from build123d import *

# Parameters (mm, degrees)
SKETCH1_W           = 40
SKETCH1_H           = 80
BOSS_EXTRUDE1_DEPTH = 100
CUT_EXTRUDE1_REACH  = 119.319
SKETCH3_W           = 40
SKETCH3_H           = 80
CUT_EXTRUDE2_REACH  = 119.319
SKETCH5_W           = 20
SKETCH5_H           = 40
CUT_EXTRUDE3_REACH  = 114.34
SKETCH6_R           = 12.5
CUT_EXTRUDE5_REACH  = 114.34


with BuildPart() as part:
    # Sketch1 → Boss-Extrude1 (new body)
    with BuildSketch(Plane(origin=(0, 0, 0), x_dir=(1, 0, 0), z_dir=(0, 1, 0))):
        with Locations((-1.364903769, -6.515993016)):
            Rectangle(SKETCH1_W, SKETCH1_H)
    extrude(amount=BOSS_EXTRUDE1_DEPTH)

    # Sketch3 → Cut-Extrude1 (cut, up to next)
    with BuildSketch(Plane(origin=(18.635096231, 0, 0), x_dir=(0, 0, -1), z_dir=(1, 0, 0)), mode=Mode.PRIVATE) as cut_extrude1_sk1:
        with Locations((-6.515993016, 60)):
            Rectangle(SKETCH3_W, SKETCH3_H)
    cut_extrude1_tool1 = extrude(cut_extrude1_sk1.sketch, amount=-CUT_EXTRUDE1_REACH, mode=Mode.PRIVATE) & part.part
    add(cut_extrude1_tool1.solids().sort_by_distance((18.635096, 60, 6.515993))[0], mode=Mode.SUBTRACT)

    # Sketch5 → Cut-Extrude2 (cut, up to next)
    with BuildSketch(Plane(origin=(18.635096231, 0, 0), x_dir=(0, 0, -1), z_dir=(1, 0, 0)), mode=Mode.PRIVATE) as cut_extrude2_sk1:
        with Locations((-36.515993016, 80)):
            Rectangle(SKETCH5_W, SKETCH5_H)
    cut_extrude2_tool1 = extrude(cut_extrude2_sk1.sketch, amount=-CUT_EXTRUDE2_REACH, mode=Mode.PRIVATE) & part.part
    add(cut_extrude2_tool1.solids().sort_by_distance((18.635096, 80, 36.515993))[0], mode=Mode.SUBTRACT)

    # Sketch6 → Cut-Extrude3 (cut, up to next)
    with BuildSketch(Plane.XZ, mode=Mode.PRIVATE) as cut_extrude3_sk1:
        with Locations((-1.364903769, 46.515993016)):
            Circle(SKETCH6_R)
    cut_extrude3_tool1 = extrude(cut_extrude3_sk1.sketch, amount=-CUT_EXTRUDE3_REACH, mode=Mode.PRIVATE) & part.part
    add(cut_extrude3_tool1.solids().sort_by_distance((-1.364904, 0, 46.515993))[0], mode=Mode.SUBTRACT)

    # Sketch10 → Cut-Extrude5 (cut, up to next)
    with BuildSketch(Plane.XZ, mode=Mode.PRIVATE) as cut_extrude5_sk1:
        Polygon((-11.364903769, -18.484006984), (8.635096231, -18.484006984), (8.635096231, -28.484006984), (3.635096231, -28.484006984), (3.635096231, -33.484006984), (-6.364903769, -33.484006984), (-6.364903769, -28.484006984), (-11.364903769, -28.484006984), align=None)
    cut_extrude5_tool1 = extrude(cut_extrude5_sk1.sketch, amount=-CUT_EXTRUDE5_REACH, mode=Mode.PRIVATE) & part.part
    add(cut_extrude5_tool1.solids().sort_by_distance((-1.364904, 0, -24.984007))[0], mode=Mode.SUBTRACT)


solid = part.part
Geometry: final body of the model. Coordinates: model frame, mm. A direction names the side the tool comes from. Give positions to 0.01 mm unless a question says otherwise; leave off trailing zeros. Order: outer loops, then holes, each group sorted by start corner. A loop starts at its lowest first (then second) coordinate and runs counter-clockwise, first axis right, second up. Notation, with made-up numbers: (-31, 0) -> (11, 0) arc R21 ccw to (11, 38) -> close; hole circle Ø11 at (14.25, -13). An arc over 180 degrees is marked (long way). Answer as a JSON object with one key per item and string values.
Q1. Section C-C (x = -10). Output: boundary loops of the cut face in (y, z), plus the area to 3 significant figures.
Entries:
{"outline": "(0, -33.48) -> (100, -33.48) -> (100, -28.48) -> (0, -28.48) -> close; (0, -18.48) -> (100, -18.48) -> (100, -13.48) -> (20, -13.48) -> (20, 26.52) -> (60, 26.52) -> (60, 37.48) -> (0, 37.48) -> close", "area": "2,460 mm^2"}
Q2. Section A-A (y = 30). Output: boundary loops of the cut face in (x, z).
Entries:
{"outline": "(-21.36, -33.48) -> (-6.36, -33.48) -> (-6.36, -28.48) -> (-11.36, -28.48) -> (-11.36, -18.48) -> (8.64, -18.48) -> (8.64, -28.48) -> (3.64, -28.48) -> (3.64, -33.48) -> (18.64, -33.48) -> (18.64, -13.48) -> (-21.36, -13.48) -> close; (-21.36, 26.52) -> (18.64, 26.52) -> (18.64, 46.52) -> (11.14, 46.52) arc R12.5 cw to (-13.86, 46.52) -> (-21.36, 46.52) -> close"}
Q3. Material intervals for probe 1 along Z at (x, y) = (-11, 89); probe 2 along Z at (x, y) = (5.5, 32); probe 3 along Z at (x, y) = (6.5, 22), sorted ascending.
Entries:
{"probe 1": "z = -33.48 to -28.48, -18.48 to -13.48", "probe 2": "z = -33.48 to -28.48, -18.48 to -13.48, 26.52 to 36.07", "probe 3": "z = -33.48 to -28.48, -18.48 to -13.48, 26.52 to 36.8"}
Q4. Access query for faces 4 (the flat face through (-1, 60, 32)), 5 (the flat face through (-1, 40, 26.516)), 6 (the flat face through (-11.365, 49, -24)). Directions: +Z, -Z, +X, -X, +Y, -Y. A direction counts if a zero-diameter tool reaches every point of the face in a straight line with its end or side. Return the directions, or none.
Entries:
{"face 4": "+Z, +X, -X, +Y", "face 5": "+X, -X, +Y", "face 6": "+Y, -Y"}
Q5. First-contact query: pin 1 (6 mm diameter, centred on x = 0, y = 56.5, fed in from -Z); pin 2 (22 mm diameter, centred on x = 2, z = 34.5, fed in from +Y); pin 3 (1 mm diameter, centred on x = 3, y = 71.5, fed in from +Z). Flat tips, straight axial feed; report the tip coordinate or a pass-through.
Entries:
{"pin 1": "stops at z = -18.48", "pin 2": "stops at y = 60", "pin 3": "stops at z = -13.48"}
Q6. Section D-D (y = 68). Output: boundary loops of the cut face in (x, z), plus the area to 3 significant figures.
Entries:
{"outline": "(-21.36, -33.48) -> (-6.36, -33.48) -> (-6.36, -28.48) -> (-11.36, -28.48) -> (-11.36, -18.48) -> (8.64, -18.48) -> (8.64, -28.48) -> (3.64, -28.48) -> (3.64, -33.48) -> (18.64, -33.48) -> (18.64, -13.48) -> (-21.36, -13.48) -> close", "area": "550 mm^2"}
Q7. Section B-B (x = 13). Output: boundary loops of the cut face in (y, z).
Entries:
{"outline": "(0, -33.48) -> (100, -33.48) -> (100, -13.48) -> (20, -13.48) -> (20, 26.52) -> (60, 26.52) -> (60, 46.52) -> (0, 46.52) -> close"}
Q8. Draft query along X for faces 1 (the flat face through (-14, 49, -33.484)), 2 (the flat face through (8.635, 49, -23)), 3 (the flat face through (-21.365, 16, -2)). Return one class per face: released by +X, released by -X, zero draft, split by the parting line, or undercut.
Entries:
{"face 1": "zero draft", "face 2": "undercut", "face 3": "released by -X"}
